The model under review builds one solid part; all positions refer to its coordinate system, in mm. A direction names the side the tool comes from. Give positions to 0.01 mm unless a question says otherwise; leave off trailing zeros. Order: outer loops, then holes, each group sorted by start corner. A loop starts at its lowest first (then second) coordinate and runs counter-clockwise, first axis right, second up. Notation, with made-up numbers: (57, 32.25) - (82, 32.25) arc R20 ccw to (82, 37.25) - close; hole circle Ø2 at (31, 72.25). An arc over 180 degrees is marked (long way). Put each result on its own line as item: value.
Autodesk Inventor part; units mm, degrees
ref_plane "YZ Plane" through (0, 0, 0) normal (1, 0, 0) x (0, 1, 0)
ref_plane "XZ Plane" through (0, 0, 0) normal (0, 1, 0) x (-1, 0, 0)
ref_plane "XY Plane" through (0, 0, 0) normal (0, 0, 1) x (1, 0, 0)
sketch "Sketch1" plane through (0, 0, 0) normal (0, 0, 1) x (1, 0, 0)
  line L0 (-12.7, -25.4) -> (12.7, -25.4)
  line L1 (12.7, -25.4) -> (12.7, 25.4)
  line L2 (12.7, 25.4) -> (-12.7, 25.4)
  line L3 (-12.7, 25.4) -> (-12.7, -25.4)
  line L4 (-12.7, -25.4) -> (12.7, 25.4) construction
  line L5 (12.7, -25.4) -> (-12.7, 25.4) construction
  line L6 (-11.1125, 23.8125) -> (11.1125, 23.8125)
  line L7 (11.1125, 23.8125) -> (11.1125, -23.8125)
  line L8 (11.1125, -23.8125) -> (-11.1125, -23.8125)
  line L9 (-11.1125, -23.8125) -> (-11.1125, 23.8125)
  point P0 (0, 0)
  dimension "width" = 25.4
  dimension "height" = 50.8
  dimension "thickness" = 1.5875
extrude "Extrusion1" add sketch "Sketch1" along normal mid plane 914.4
properties part number "MU-EV-01" material "Aluminum 6061"
(1) The part is to be moulded in two halves that separate along Y. For faces 3 (the flat face through (-11.3, 2, 457.2)), 4 (the flat face through (0, 25.4, -6)), 5 (the flat face through (0, 23.812, -6)), say which applies: pulls with the +Y half, pulls with the -Y half, needs draft (parallel to the pull), parting line crosses it, or undercut.
The answers:
face 3: needs draft
face 4: pulls with the +Y half
face 5: undercut
(2) Wall thickness on L1, parallel to X at y = 14.5, z = -231.5; L2, parallel to Y at x = 7.75, z = -340.5: over which ranges is each line inside the solid? List them lowest first.
The answers:
L1: -12.7 to -11.11, 11.11 to 12.7
L2: -25.4 to -23.81, 23.81 to 25.4
(3) For faces 1 (the flat face through (-11.112, 0, -6)), 2 (the flat face through (-12.7, 0, -6)), list the 3-axis set-ups (+Z, -Z, +X, -X, +Y, -Y) from which the entire face can be reached by the end or side of a thin tool; tool diameter is ignored.
The answers:
face 1: +Z, -Z
face 2: +Z, -Z, -X, +Y, -Y
(4) Take a section at A-A, the plane y = -11. Write out the cut boundary in (x, z), then the cut area to 3 significant figures.
The answers:
outline: (-12.7, -457.2) - (-11.11, -457.2) - (-11.11, 457.2) - (-12.7, 457.2) - close; (11.11, -457.2) - (12.7, -457.2) - (12.7, 457.2) - (11.11, 457.2) - close
area: 2,900 mm^2
(5) Take a section at C-C, the plane z = -225.5. Write out the cut boundary in (x, y).
The answers:
outline: (-12.7, -25.4) - (12.7, -25.4) - (12.7, 25.4) - (-12.7, 25.4) - close; hole (-11.11, -23.81) - (11.11, -23.81) - (11.11, 23.81) - (-11.11, 23.81) - close
(6) Take a section at B-B, the plane x = -7. Write out the cut boundary in (y, z), then the cut area to 3 significant figures.
The answers:
outline: (-25.4, -457.2) - (-23.81, -457.2) - (-23.81, 457.2) - (-25.4, 457.2) - close; (23.81, -457.2) - (25.4, -457.2) - (25.4, 457.2) - (23.81, 457.2) - close
area: 2,900 mm^2
